```python
from build123d import *

# Parameters (mm, degrees)
SKETCH1_R                  = 2
SCREW_SECTION_DEPTH        = 18
SKETCH2_R                  = 3.5
BAR_SECTION_DEPTH          = 21.5
MOUNT_SECTION_DEPTH        = 1.6
BAR_TAPER_DEPTH            = 6
MOUNT_FILLET_R             = 0.5
MOUNT_FILLET_OF_MIRROR_2_R = 0.5


with BuildPart() as part:
    # Sketch1 → Screw Section (new body)
    with BuildSketch(Plane.XY):
        Circle(SKETCH1_R)
    screw_section = extrude(amount=SCREW_SECTION_DEPTH)

    # Sketch2 → Bar Section (add)
    with BuildSketch(Plane.XY.offset(18)):
        Circle(SKETCH2_R)
    bar_section = extrude(amount=BAR_SECTION_DEPTH)

    # Sketch3 → Mount Section (add, symmetric)
    with BuildSketch(Plane(origin=(0, 0, 0), x_dir=(1, 0, 0), z_dir=(0, 1, 0))):
        with BuildLine():
            Line((5, -39.5), (-5, -39.5))
            Line((-5, -39.5), (-5, -44.5))
            ThreePointArc((-5, -44.5), (0, -49.5), (5, -44.5))
            Line((5, -44.5), (5, -39.5))
        make_face()
    mount_section = extrude(amount=MOUNT_SECTION_DEPTH, both=True)

    # Sketch4 → Bar Taper (cut, symmetric)
    with BuildSketch(Plane(origin=(0, 0, 0), x_dir=(0, 0, -1), z_dir=(1, 0, 0))):
        Polygon((-34.5, -3.5), (-39.5, -1.6), (-39.5, -3.5), align=None)
        Polygon((-34.5, 3.5), (-39.5, 1.6), (-39.5, 3.5), align=None)
    bar_taper = extrude(amount=BAR_TAPER_DEPTH, both=True, mode=Mode.SUBTRACT)

    # Mount Fillet
    mount_fillet_edges = [part.edges().sort_by_distance(p)[0] for p in [
        (-5, 0, 39.5),
        (3.401842713, -0.823083322, 39.5),
        (-3.5, 0, 39.5),
        (5, 0, 39.5),
    ]]
    fillet(mount_fillet_edges, radius=MOUNT_FILLET_R)

    # Sketch6 → Ball Hole (revolve, cut)
    with BuildSketch(Plane(origin=(0, 0, 0), x_dir=(0, 0, -1), z_dir=(1, 0, 0))):
        with BuildLine():
            Line((-46.420937271, -1.6), (-44.5, -1.6))
            Line((-44.5, -1.6), (-44.5, 1.6))
            Line((-44.5, 1.6), (-46.420937271, 1.6))
            ThreePointArc((-46.420937271, 1.6), (-47, 0), (-46.420937271, -1.6))
        make_face()
    ball_hole = revolve(axis=Axis((0, -1.6, 44.5), (0, 1, 0)), mode=Mode.SUBTRACT)

    # Mirror 2: Screw Section, Bar Section, Mount Section, Bar Taper, Ball Hole across Front Plane
    add(screw_section.mirror(Plane.XY))
    add(bar_section.mirror(Plane.XY))
    add(mount_section.mirror(Plane.XY))
    add(bar_taper.mirror(Plane.XY), mode=Mode.SUBTRACT)
    add(ball_hole.mirror(Plane.XY), mode=Mode.SUBTRACT)

    # Mount Fillet of Mirror 2
    mount_fillet_of_mirror_2_edges = [part.edges().sort_by_distance(p)[0] for p in [
        (-5, 0, -39.5),
        (3.401842713, -0.823083322, -39.5),
        (-3.5, 0, -39.5),
        (5, 0, -39.5),
    ]]
    fillet(mount_fillet_of_mirror_2_edges, radius=MOUNT_FILLET_OF_MIRROR_2_R)


solid = part.part
```
Geometry check sheet. Reference: the model listing, model coordinates, mm. A direction names the side the tool comes from. Give positions to 0.01 mm unless a question says otherwise; leave off trailing zeros. Order: outer loops, then holes, each group sorted by start corner. A loop starts at its lowest first (then second) coordinate and runs counter-clockwise, first axis right, second up. Notation, with made-up numbers: (41, 47) - (76, 47) arc R19 cw to (76, 60) - close; hole circle Ø11 at (-20.75, -31). An arc over 180 degrees is marked (long way). Write item = value, one per line. Start each with the question number.
1) Scan lines: L1, parallel to Y at x = 0.25, z = 15.5; L2, parallel to X at y = 3, z = 29.5; L3, parallel to Z at x = 3.5, y = -1.5. Record each from-to range of solid material in increasing order.
2) Section check C-C (z = 7). Enter the section's corners in (x, y), then the cut area to 3 significant figures.
3) Section check B-B (x = 0). Enter the section's corners in (y, z).
4) Draft check along Z on faces 1 (the cylindrical face through (0, -2, 0)), 2 (the flat face through (0, -1.6, 42)), 3 (the flat face through (0.051, 2.352, 37.521)), 4 (the cylindrical face through (1.615, -3.105, -28.353)). Enter one of: released by +Z, released by -Z, zero draft, split by the parting line, or undercut.
5) Access from +Z, -Z, +X, -X, +Y, -Y to the whole of each face (thin tool, end or side, straight path). Record for faces 5 (the cylindrical face through (1.615, -3.105, 28.353)), 6 (the flat face through (0, 1.6, 42)), 7 (the flat face through (0, -1.6, -42)).
6) Section check A-A (y = 0). Count the separate pieces of the cut face and the enclosed holes in it, then the cut area to 3 significant figures.
7) Gauge pin test, flat ends, axial feed: pin 1 Ø1 at (y, z) = (2, -20) entering from -X; pin 2 Ø6 at (x, z) = (-4, 2) entering from -Y; pin 3 Ø0.7 at (x, y) = (-4, 0.5) entering from -Z. Record the tip position at first contact, or that the pin passes through.
8) Section check D-D (z = -28). Enter the section's corners in (x, y), then the cut area to 3 significant figures.
Geometry check:
q1.L1 = -1.98 to 1.98
q1.L2 = -1.8 to 1.8
q1.L3 = -48.07 to -39.46, 39.46 to 48.07
q2.outline = circle Ø4 at (0, 0)
q2.area = 12.6 mm2
q3.outline = (-3.5, -34.5) - (-1.6, -39.5) - (-1.6, -42.58) arc R2.5 cw to (1.6, -42.58) - (1.6, -39.5) - (3.5, -34.5) - (3.5, -18) - (2, -18) - (2, 18) - (3.5, 18) - (3.5, 34.5) - (1.6, 39.5) - (1.6, 42.58) arc R2.5 cw to (-1.6, 42.58) - (-1.6, 39.5) - (-3.5, 34.5) - (-3.5, 18) - (-2, 18) - (-2, -18) - (-3.5, -18) - close; (-1.6, -49.5) - (1.6, -49.5) - (1.6, -46.42) arc R2.5 cw to (-1.6, -46.42) - close; (-1.6, 46.42) arc R2.5 cw to (1.6, 46.42) - (1.6, 49.5) - (-1.6, 49.5) - close
q4.face_1 = undercut
q4.face_2 = zero draft
q4.face_3 = released by +Z
q4.face_4 = undercut
q5.face_5 = none
q5.face_6 = +Z, +X, -X, +Y
q5.face_7 = -Z, +X, -X, -Y
q6.separate_pieces = 1
q6.enclosed_holes = 2
q6.area = 584 mm2
q7.pin_1 = -3.16
q7.pin_2 = -1.73
q7.pin_3 = -47.92
q8.outline = circle Ø7 at (0, 0)
q8.area = 38.5 mm2
